Read the model definition and answer for the solid it produces. Units are mm, in the model's axes. Coordinates: 2 decimals unless noted, no trailing zeros. Write each loop counter-clockwise with the first axis right and the second up, starting at its lowest first coordinate (ties: lowest second). Pieces come first, ordered by that corner, then holes. Notation, with made-up numbers: (49.5, 16.5) -> (94.5, 16.5) arc R17 ccw to (94.5, 29.5) -> close; hole circle Ø6 at (77, 74.25). An arc over 180 degrees is marked (long way). Write item = value, one per line. Start each with the question number.
1) Flat-ended cylindrical pins translate along their axes: pin 1 Ø3 at (x, z) = (923, -1.5) entering from +Y; pin 2 Ø1.5 at (y, z) = (-1019, -3.5) entering from +X. Find the tip coordinate at first contact, or state that the pin passes through.
2) Section A-A (z = -2.65) is taken. Determine the outline of the cut face in (x, y), plus the area to 3 significant figures.
3) Find the intervals of material crossed by line 1 along Y through (x, z) = (601.5, -1.15); line 2 along X through (y, z) = (-1160.5, -0.7), in increasing order. Write a range as from..to.
4) Section B-B (y = -1279) is taken. Determine the outline of the cut face in (x, z), plus the area to 4 significant figures.
5) Section C-C (x = 835) is taken. Determine the outline of the cut face in (y, z), plus the area to 3 significant figures.
from build123d import *

# Parameters (mm, degrees)
TABAN_FLAN_1_DEPTH         = 5
KES_EKSTR_ZYON1_DEPTH      = 2347.284296499
KES_EKSTR_ZYON1_DEPTH_BACK = 2347.284296499


# Sheet-metal steps are written as plain solids
with BuildPart() as part:
    # Çizim1 → Taban-Flanş1 (new body)
    with BuildSketch(Plane.XY):
        Polygon((0, 0), (1195, 0), (1195, -895), (1800, -895), (1800, -1505), (0, -1505), align=None)
    extrude(amount=-TABAN_FLAN_1_DEPTH)

    # Çizim2 → Kes-Ekstrüzyon1 (cut, two sides: drawn at the far end of the back side and taken through both)
    with BuildSketch(Plane.XY.offset(-KES_EKSTR_ZYON1_DEPTH_BACK)):
        Polygon((525, -1505), (525, -830), (1195, -830), (1965.528313332, -849.744695172), (1943.261334952, -1718.704035599), align=None)
    extrude(amount=KES_EKSTR_ZYON1_DEPTH + KES_EKSTR_ZYON1_DEPTH_BACK, mode=Mode.SUBTRACT)


solid = part.part
Answer key:
q1.pin_1 = 0
q1.pin_2 = 525
q2.outline = (0, -1505) -> (525, -1505) -> (525, -830) -> (1195, -830) -> (1195, 0) -> (0, 0) -> close
q2.area = 1,350,000 mm^2
q3.line_1 = -830..0
q3.line_2 = 0..525
q4.outline = (0, -5) -> (525, -5) -> (525, 0) -> (0, 0) -> close
q4.area = 2,625 mm^2
q5.outline = (-830, -5) -> (0, -5) -> (0, 0) -> (-830, 0) -> close
q5.area = 4,150 mm^2
